```python
from build123d import *

# Parameters (mm, degrees)
F0_W          = 4
F0_H          = 8
F0_H_2        = 2
F0_W_2        = 5.5
F0_H_3        = 3.5
F0_W_3        = 4.25
F0_H_4        = 26
F1_DEPTH      = 8
F2_R          = 3.99999
F3_T1_DEPTH   = 37.8956518578
F4_T1_DEPTH   = 21.1532650868
F5_T1_DEPTH   = 21.1532650868
F6_R          = 1.75
F7_DEPTH      = 10
F8_T1_DEPTH   = 32.4948974279
F9_R          = 7
F10_R         = 10
F11_T1_DEPTH  = 8
F12_R         = 3
F13_T1_DEPTH  = 8
F13_T3_DEPTH  = 8
F13_T5_DEPTH  = 8
F13_T7_DEPTH  = 8
F13_T9_DEPTH  = 8
F13_T11_DEPTH = 8
F13_T13_DEPTH = 8
F13_T15_DEPTH = 8
F13_T17_DEPTH = 8
F13_T19_DEPTH = 8
F13_T21_DEPTH = 13
F13_T23_DEPTH = 13


# Not quite as in the source:
# - a fillet or chamfer that OpenCascade refuses, or shapes differently, is made with other operations: its cross-section is extruded or revolved along the edge and cut away or added
# - two fillets or chamfers of one size are made in one step
# - a fillet or chamfer is up to 0.001 mm smaller than in the source, because OpenCascade refuses the exact size


with BuildPart() as f1:
    # F0 (on Top) → F1 (new body)
    with BuildSketch(Plane.XY):
        Polygon((0, 83), (0, 0), (11, 0), (11, 10), (11, 18.5), (6, 18.5), (6, 31.5), (8, 31.5), (11, 31.5), (13, 31.5), (13, 25.5), (17, 25.5), (17, 28.5), (17, 54.5), (17, 57.5), (13, 57.5), (13, 51.5), (11, 51.5), (8, 51.5), (6, 51.5), (6, 64.5), (11, 64.5), (11, 73), (11, 83), align=None)
        with Locations((22, 68.5)):
            Rectangle(F0_W, F0_H)
        with Locations((22, 63.5)):
            Rectangle(F0_W, F0_H_2)
        with Locations((21.25, 57.75)):
            Rectangle(F0_W_2, F0_H_3)
        with Locations((21.25, 25.25)):
            Rectangle(F0_W_2, F0_H_3)
        with Locations((22, 19.5)):
            Rectangle(F0_W, F0_H_2)
        with Locations((22, 14.5)):
            Rectangle(F0_W, F0_H)
        Polygon((11, 23.5), (11, 20.5), (20, 20.5), (24, 20.5), (24, 23.5), (18.5, 23.5), (17, 23.5), align=None)
        Polygon((8, 20.5), (11, 20.5), (11, 23.5), (11, 25.5), (11, 31.5), (8, 31.5), align=None)
        Polygon((11, 59.5), (11, 62.5), (8, 62.5), (8, 51.5), (11, 51.5), (11, 57.5), align=None)
        Polygon((20, 62.5), (11, 62.5), (11, 59.5), (17, 59.5), (18.5, 59.5), (24, 59.5), (24, 62.5), align=None)
        with Locations((19.125, 41.5)):
            Rectangle(F0_W_3, F0_H_4)
    extrude(amount=F1_DEPTH)

    # F2 (radius 4 in the source; OpenCascade refuses exactly that, so slightly less here)
    f2_edges = [f1.edges().sort_by_distance(p)[0] for p in [
        (5.5, 83, 8),
        (5.5, 0, 8),
        (5.5, 0, 0),
        (5.5, 83, 0),
    ]]
    fillet(f2_edges, radius=F2_R)

    # F3: fillet of radius 6 on 2 edges, made by hand

    # F3_s2 → F3_t1 (cut)
    with BuildSketch(Plane.XY.offset(-14.9478259289)):
        with BuildLine():
            ThreePointArc((24, 61.9791303716), (22.4158804332, 57.9171111692), (18.5, 56))
            Line((18.5, 56), (24, 56))
            Line((24, 56), (24, 61.9791303716))
        make_face()
        with BuildLine():
            ThreePointArc((24, 21.0208696284), (22.4158804332, 25.0828888308), (18.5, 27))
            Line((18.5, 27), (24, 27))
            Line((24, 27), (24, 21.0208696284))
        make_face()
    extrude(amount=F3_T1_DEPTH, mode=Mode.SUBTRACT)

    # F4: chamfer of 0.5 x 2.5 on 1 edges, made by hand

    # F4_s2 → F4_t1 (cut)
    with BuildSketch(Plane.XY.offset(-6.5766325434)):
        with BuildLine():
            Line((19.379363756, 56.0377654524), (18.466798813, 58.6304434947))
            Line((18.466798813, 58.6304434947), (18.416798813, 58.6304434947))
            ThreePointArc((18.416798813, 58.6304434947), (18.45, 57.3152217474), (18.45, 56))
            Line((18.45, 56), (18.5041666667, 55.9501739136))
            ThreePointArc((18.5041666667, 55.9501739136), (18.9421943049, 56.0029468158), (19.3905817774, 55.9890401407))
            Line((19.3905817774, 55.9890401407), (19.379363756, 56.0377654524))
        make_face()
    extrude(amount=F4_T1_DEPTH, mode=Mode.SUBTRACT)

    # F5: chamfer of 0.5 x 2.5 on 1 edges, made by hand

    # F5_s2 → F5_t1 (cut)
    with BuildSketch(Plane.XY.offset(-6.5766325434)):
        with BuildLine():
            Line((18.466798813, 24.3695565053), (19.379363756, 26.9622345476))
            Line((19.379363756, 26.9622345476), (19.3905817774, 27.0109598593))
            ThreePointArc((19.3905817774, 27.0109598593), (18.9421943049, 26.9970531842), (18.5041666667, 27.0498260864))
            Line((18.5041666667, 27.0498260864), (18.45, 27))
            ThreePointArc((18.45, 27), (18.45, 25.6847782526), (18.416798813, 24.3695565053))
            Line((18.416798813, 24.3695565053), (18.466798813, 24.3695565053))
        make_face()
    extrude(amount=F5_T1_DEPTH, mode=Mode.SUBTRACT)

    # F6 (on face) → F7 (cut)
    with BuildSketch(Plane(origin=(0, 0, 0), x_dir=(0, -1, 0), z_dir=(-1, 0, 0))):
        with Locations((-79, 4)):
            Circle(F6_R)
        with Locations((-4, 4)):
            Circle(F6_R)
    extrude(amount=-F7_DEPTH, mode=Mode.SUBTRACT)

    # F8: fillet of radius 5 on 2 edges, made by hand

    # F8_s2 → F8_t1 (cut)
    with BuildSketch(Plane.XY.offset(-12.2474487139)):
        with BuildLine():
            ThreePointArc((13, 52.6010205144), (14.1270166538, 55.7632981746), (17, 57.5))
            Line((17, 57.5), (13, 57.5))
            Line((13, 57.5), (13, 52.6010205144))
        make_face()
        with BuildLine():
            ThreePointArc((17, 25.5), (14.1270166538, 27.2367018254), (13, 30.3989794856))
            Line((13, 30.3989794856), (13, 25.5))
            Line((13, 25.5), (17, 25.5))
        make_face()
    extrude(amount=F8_T1_DEPTH, mode=Mode.SUBTRACT)

    # F9
    f9_edges = [f1.edges().sort_by_distance(p)[0] for p in [
        (11, 59.5, 4),
        (11, 23.5, 4),
    ]]
    fillet(f9_edges, radius=F9_R)

    # F10
    f10_edges = [f1.edges().sort_by_distance(p)[0] for p in [
        (8, 62.5, 4),
        (8, 20.5, 4),
    ]]
    fillet(f10_edges, radius=F10_R)

    # F11: fillet of radius 12 on 2 edges, made by hand

    # F11_s2 → F11_t1 (join)
    with BuildSketch(Plane.XY):
        with BuildLine():
            ThreePointArc((6, 54.7532056552), (7.322921748, 60.2304312302), (11, 64.5))
            Line((11, 64.5), (6, 64.5))
            Line((6, 64.5), (6, 54.7532056552))
        make_face()
        with BuildLine():
            ThreePointArc((11, 18.5), (7.322921748, 22.7695687698), (6, 28.2467943448))
            Line((6, 28.2467943448), (6, 18.5))
            Line((6, 18.5), (11, 18.5))
        make_face()
    extrude(amount=F11_T1_DEPTH)

    # F12
    f12_edges = [f1.edges().sort_by_distance(p)[0] for p in [
        (20, 62.5, 4),
        (20, 20.5, 4),
    ]]
    fillet(f12_edges, radius=F12_R)

    # F13: fillet of radius 1 on 12 edges, made by hand

    # F13_s2 → F13_t1 (join)
    with BuildSketch(Plane.XY):
        with BuildLine():
            ThreePointArc((8, 52.5), (7.7071067812, 51.7928932188), (7, 51.5))
            Line((7, 51.5), (8, 51.5))
            Line((8, 51.5), (8, 52.5))
        make_face()
    extrude(amount=F13_T1_DEPTH)

    # F13_s4 → F13_t3 (join)
    with BuildSketch(Plane.XY):
        with BuildLine():
            ThreePointArc((7, 51.5), (6.2928932188, 51.7928932188), (6, 52.5))
            Line((6, 52.5), (6, 51.5))
            Line((6, 51.5), (7, 51.5))
        make_face()
    extrude(amount=F13_T3_DEPTH)

    # F13_s6 → F13_t5 (join)
    with BuildSketch(Plane.XY):
        with BuildLine():
            ThreePointArc((18.5, 58.536115974), (18.1575199019, 59.2341109303), (17.4185535189, 59.4758096297))
            Line((17.4185535189, 59.4758096297), (17.4102471406, 59.575464053))
            ThreePointArc((17.4102471406, 59.575464053), (18, 59.6), (18.5, 59.6))
            Line((18.5, 59.6), (18.6, 59.5))
            ThreePointArc((18.6, 59.5), (18.6, 59.018057987), (18.5998382698, 58.5418010318))
            Line((18.5998382698, 58.5418010318), (18.5, 58.536115974))
        make_face()
    extrude(amount=F13_T5_DEPTH)

    # F13_s8 → F13_t7 (join)
    with BuildSketch(Plane.XY):
        with BuildLine():
            ThreePointArc((11, 52.5), (11.2928932188, 51.7928932188), (12, 51.5))
            Line((12, 51.5), (11, 51.5))
            Line((11, 51.5), (11, 52.5))
        make_face()
    extrude(amount=F13_T7_DEPTH)

    # F13_s10 → F13_t9 (join)
    with BuildSketch(Plane.XY):
        with BuildLine():
            ThreePointArc((13, 52.5), (12.7071067812, 51.7928932188), (12, 51.5))
            Line((12, 51.5), (13, 51.5))
            Line((13, 51.5), (13, 52.5))
        make_face()
    extrude(amount=F13_T9_DEPTH)

    # F13_s12 → F13_t11 (join)
    with BuildSketch(Plane.XY):
        with BuildLine():
            ThreePointArc((7, 31.5), (6.2928932188, 31.2071067812), (6, 30.5))
            Line((6, 30.5), (6, 31.5))
            Line((6, 31.5), (7, 31.5))
        make_face()
    extrude(amount=F13_T11_DEPTH)

    # F13_s14 → F13_t13 (join)
    with BuildSketch(Plane.XY):
        with BuildLine():
            ThreePointArc((7, 31.5), (7.7071067812, 31.2071067812), (8, 30.5))
            Line((8, 30.5), (8, 31.5))
            Line((8, 31.5), (7, 31.5))
        make_face()
    extrude(amount=F13_T13_DEPTH)

    # F13_s16 → F13_t15 (join)
    with BuildSketch(Plane.XY):
        with BuildLine():
            ThreePointArc((13, 30.5), (12.7071067812, 31.2071067812), (12, 31.5))
            Line((12, 31.5), (13, 31.5))
            Line((13, 31.5), (13, 30.5))
        make_face()
    extrude(amount=F13_T15_DEPTH)

    # F13_s18 → F13_t17 (join)
    with BuildSketch(Plane.XY):
        with BuildLine():
            ThreePointArc((11, 30.5), (11.2928932188, 31.2071067812), (12, 31.5))
            Line((12, 31.5), (11, 31.5))
            Line((11, 31.5), (11, 30.5))
        make_face()
    extrude(amount=F13_T17_DEPTH)

    # F13_s20 → F13_t19 (join)
    with BuildSketch(Plane.XY):
        with BuildLine():
            ThreePointArc((17.4185535189, 23.5241903703), (18.1575199019, 23.7658890697), (18.5, 24.463884026))
            Line((18.5, 24.463884026), (18.5998382698, 24.4581989682))
            ThreePointArc((18.5998382698, 24.4581989682), (18.6, 23.981942013), (18.6, 23.5))
            Line((18.6, 23.5), (18.5, 23.4))
            ThreePointArc((18.5, 23.4), (18, 23.4), (17.4102471406, 23.424535947))
            Line((17.4102471406, 23.424535947), (17.4185535189, 23.5241903703))
        make_face()
    extrude(amount=F13_T19_DEPTH)

    # F13_s22 → F13_t21 (cut)
    with BuildSketch(Plane.XY.offset(-2.5)):
        with BuildLine():
            ThreePointArc((20.25, 54.5), (20.9571067812, 54.2071067812), (21.25, 53.5))
            Line((21.25, 53.5), (21.25, 54.5))
            Line((21.25, 54.5), (20.25, 54.5))
        make_face()
    extrude(amount=F13_T21_DEPTH, mode=Mode.SUBTRACT)

    # F13_s24 → F13_t23 (cut)
    with BuildSketch(Plane.XY.offset(-2.5)):
        with BuildLine():
            ThreePointArc((21.25, 29.5), (20.9571067812, 28.7928932188), (20.25, 28.5))
            Line((20.25, 28.5), (21.25, 28.5))
            Line((21.25, 28.5), (21.25, 29.5))
        make_face()
    extrude(amount=F13_T23_DEPTH, mode=Mode.SUBTRACT)


solid = f1.part
```
Design review of the part built by this model. Coordinates are the model's own, in mm. A direction names the side the tool comes from. Round coordinates to 2 decimals unless told otherwise and drop trailing zeros. Write each loop counter-clockwise with the first axis right and the second up, starting at its lowest first coordinate (ties: lowest second). Pieces come first, ordered by that corner, then holes.
Item 1: Clearance check with flat-ended pins moving along their axes: pin 1 Ø4 at (y, z) = (78.5, 4.5) entering from -X; pin 2 Ø2.5 at (x, z) = (19.5, 4) entering from -Y; pin 3 Ø1.5 at (x, z) = (6, 6) entering from +Y; pin 4 Ø2 at (y, z) = (79, 4) entering from -X. State where each tip first meets the part, or that it passes through.
Item 2: We need section B-B on x = 4.25. State how many separate pieces and enclosed holes the cut face has, and give its area (3 significant figures).
Item 3: We need section D-D on x = 13.75. Write out the cut boundary in (y, z), and give its area (3 significant figures).
Item 4: For faces 5 (the cylindrical face through (12.8, 25.814, 4.056)), 6 (the flat face through (19, 54.5, 4)), 7 (the flat face through (22, 10.5, 4)), 8 (the cylindrical face through (4.93, 77.331, 4.526)), list the 3-axis set-ups (+Z, -Z, +X, -X, +Y, -Y) from which the entire face can be reached by the end or side of a thin tool; tool diameter is ignored.
Item 5: We need section A-A on y = 13. Write out the cut boundary in (x, z), and give its area (3 significant figures).
Item 6: We need section C-C on x = 22. Write out the cut boundary in (y, z).
Item 7: For probe 1 along X at (y, z) = (29.5, 7.5); probe 2 along Y at (x, z) = (12.5, 2.5); probe 3 along Z at (x, y) = (3, 79), list the stretches that pass through material, from the lowest coordinate up.
Item 8: The part is to be moulded in two halves that separate along Z. For faces 1 (the flat face through (10, 42, 0)), 2 (the cylindrical face through (7.287, 60.159, 3.944)), 3 (the flat face through (10, 79, 4)), 4 (the cylindrical face through (5.577, 1.141, 6.797)), say which applies: +Z half, -Z half, draft (parallel to the pull), parting line (faces both ways), or undercut.
Returned:
1. pin 1: stops at x = 0
1. pin 2: stops at y = 10.5
1. pin 3: stops at y = 82.8
1. pin 4: stops at x = 10
2. separate pieces: 1
2. enclosed holes: 2
2. area: 631 mm2
3. outline: (21.45, 0) - (24.94, 0) - (24.94, 8) - (21.45, 8) - close; (27.77, 0) - (55.23, 0) - (55.23, 8) - (27.77, 8) - close; (58.06, 0) - (61.55, 0) - (61.55, 8) - (58.06, 8) - close
3. area: 276 mm2
4. face 5: +Z, -Z
4. face 6: +Z, -Z, +X
4. face 7: +Z, -Z, +X, -Y
4. face 8: -X
5. outline: (0, 0) - (11, 0) - (11, 8) - (0, 8) - close; (20, 0) - (24, 0) - (24, 8) - (20, 8) - close
5. area: 120 mm2
6. outline: (10.5, 0) - (25.49, 0) - (25.49, 8) - (10.5, 8) - close; (57.51, 0) - (72.5, 0) - (72.5, 8) - (57.51, 8) - close
7. probe 1: x = 0 to 6, 8.05 to 11.07, 13.08 to 21.25
7. probe 2: y = 22.15 to 26.17, 31.37 to 51.63, 56.83 to 60.85
7. probe 3: z = 0 to 2.25, 5.75 to 8
8. face 1: -Z half
8. face 2: draft
8. face 3: undercut
8. face 4: +Z half
